Build history of the part. All positions in model axes, mm. Round coordinates to 2 decimals unless told otherwise and drop trailing zeros. Loops run counter-clockwise (first coordinate to the right, second up) from the corner with the lowest first, then second, coordinate; pieces in that order, holes last. Notation, with made-up numbers: (-15.5, 62.5) - (25.5, 62.5) arc R25 cw to (25.5, 80.5) - close; hole circle Ø3 at (5.25, 78.25). An arc over 180 degrees is marked (long way). One line per question, with ' | ' between items. Start each with the question number.
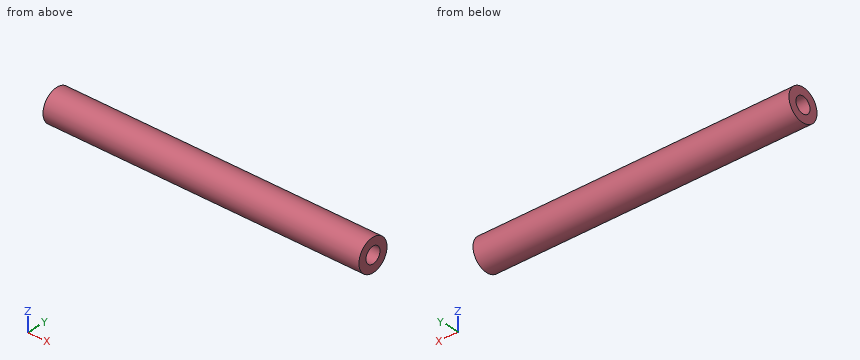
from build123d import *

# Parameters (mm, degrees)
SKETCH1_R           = 6.35
BOSS_EXTRUDE1_DEPTH = 63.5
SKETCH2_R           = 3.175
CUT_EXTRUDE1_DEPTH  = 128.317104114
SCALE1_SCALE        = 0.5


with BuildPart() as part:
    # Sketch1 → Boss-Extrude1 (new, symmetric)
    with BuildSketch(Plane(origin=(0, 0, 0), x_dir=(0, 0, -1), z_dir=(1, 0, 0))):
        Circle(SKETCH1_R)
    extrude(amount=BOSS_EXTRUDE1_DEPTH, both=True)

    # Sketch2 → Cut-Extrude1 (cut, through all)
    with BuildSketch(Plane(origin=(63.5, 0, 0), x_dir=(0, 0, -1), z_dir=(1, 0, 0))):
        Circle(SKETCH2_R)
    extrude(amount=-CUT_EXTRUDE1_DEPTH, mode=Mode.SUBTRACT)


with BuildPart() as part_1:
    # Scale1: scaled about (0, 0, 0)
    add(part.part.scale(SCALE1_SCALE))


solid = part_1.part
1) Wall check: line 1 (Y direction, x = -5.5, z = 0) (1 decimal); line 2 (Z direction, x = 8, y = -1); line 3 (Z direction, x = -1.5, y = 0.75). Give the ranges that are in metal, low to high. Write a range as [from, to].
2) Saw through at D-D on z = -2.5. Write the cut outline in (x, y).
3) Drop a flat-ended pin along its axis: pin 1 (1.5 mm diameter, centred on x = -20, z = -2, fed in from -Y). Give the stop position or say it passes through.
Answer key:
1) line 1: [-3.2, -1.6], [1.6, 3.2] | line 2: [-3.01, -1.23], [1.23, 3.01] | line 3: [-3.09, -1.4], [1.4, 3.09]
2) outline: (-31.75, -1.96) - (31.75, -1.96) - (31.75, 1.96) - (-31.75, 1.96) - close
3) pin 1: y = -2.92
